Verification items for the finished model (mm, model axes). A direction names the side the tool comes from. Coordinates: 2 decimals unless noted, no trailing zeros. Order: outer loops, then holes, each group sorted by start corner. A loop starts at its lowest first (then second) coordinate and runs counter-clockwise, first axis right, second up. Notation, with made-up numbers: M 9,7 L 41,7 A10 cw 41,22 Z; hole C -22.75,-21.5 d5. An arc over 180 degrees is marked long. Write item = value, one per line.
```python
from build123d import *

# Parameters (mm, degrees)
CHAMFER1_SIZE      = 1
CHAMFER2_SIZE      = 2
SKETCH2_OUTSIDE_W  = 33.844
SKETCH2_OUTSIDE_H  = 33.844
CUT_EXTRUDE1_DEPTH = 6


with BuildPart() as part:
    # Sketch1 → Revolve1 (revolve)
    with BuildSketch(Plane.XY, mode=Mode.PRIVATE) as revolve1_sk:
        with BuildLine():
            Line((87, 0), (87, 3))
            Line((87, 3), (79, 3))
            Line((79, 3), (79, 5))
            Line((79, 5), (25, 5))
            Line((25, 5), (25, 7))
            Line((25, 7), (13, 7))
            Line((13, 7), (13, 5))
            Line((13, 5), (10, 5))
            Line((10, 5), (10, 4))
            Line((10, 4), (3, 4))
            Line((3, 4), (3, 5))
            Line((3, 5), (1.310723572, 5))
            ThreePointArc((1.310723572, 5), (0.382949383, 2.571411472), (0, 0))
            Line((0, 0), (87, 0))
        make_face()
    revolve(revolve1_sk.sketch.rotate(Axis((0, 0, 0), (1, 0, 0)), 90), axis=Axis((0, 0, 0), (1, 0, 0)))

    # Chamfer1
    chamfer1_edges = [part.edges().sort_by_distance(p)[0] for p in [
        (87, 0, -3),
    ]]
    chamfer(chamfer1_edges, length=CHAMFER1_SIZE)

    # Chamfer2
    chamfer2_edges = [part.edges().sort_by_distance(p)[0] for p in [
        (13, 0, -7),
        (25, 0, -5),
    ]]
    chamfer(chamfer2_edges, length=CHAMFER2_SIZE - 0.0001)  # a hair under: the kernel refuses the full size

    # Sketch2 outside → Cut-Extrude1 (cut)
    with BuildSketch(Plane(origin=(79, 0, 0), x_dir=(0, 0, -1), z_dir=(1, 0, 0))):
        Rectangle(SKETCH2_OUTSIDE_W, SKETCH2_OUTSIDE_H)
        Polygon((0, 5.656854249), (5.656854249, 0), (0, -5.656854249), (-5.656854249, 0), align=None, mode=Mode.SUBTRACT)
    extrude(amount=-CUT_EXTRUDE1_DEPTH, mode=Mode.SUBTRACT)


solid = part.part
```
Item 1: Sectioned sample at B-B, the plane x = 82. Enter the section's corners in (y, z).
Report:
outline = C 0,0 d6
Item 2: Scan lines: L1, parallel to Z at x = 34, y = -0.75; L2, parallel to Y at x = 9.5, z = 0; L3, parallel to X at y = -1.75, z = -4. Record each from-to range of solid material in increasing order. Write a range as from..to.
Report:
L1 = -4.94..4.94
L2 = -4..4
L3 = 1.01..3, 10..73
Item 3: Tool access check on faces 1 (the flat face through (76.042, -2.799, -2.858)), 2 (the cylindrical face through (2, 0, -5)), 3 (the flat face through (73, 3, 3)). Record the directions out of +Z, -Z, +X, -X, +Y, -Y that give a thin tool (end or side, any length) a straight path to the whole face; none if there is none.
Report:
face_1 = -Z, +X, -Y
face_2 = -X
face_3 = +Z, +X, +Y
Item 4: Sectioned sample at A-A, the plane x = 72. Enter the section's corners in (y, z), then the cut area to 3 significant figures.
Report:
outline = C 0,0 d10
area = 78.5 mm^2
Item 5: Release check for a two-part mould opening along X. For faces 4 (the cylindrical face through (6.451, 3.905, -0.867)), 5 (the flat face through (79, 3.3, 0.1)), 6 (the cylindrical face through (19.93, 6.21, 3.23)) record: pulls with the +X half, pulls with the -X half, needs draft (parallel to the pull), parting line crosses it, or undercut.
Report:
face_4 = undercut
face_5 = pulls with the +X half
face_6 = needs draft
Item 6: Gauge pin test, flat ends, axial feed: pin 1 (1 mm diameter, centred on x = 61.5, z = -3.5, fed in from -Y); pin 2 (2 mm diameter, centred on y = -2, z = 3.5, fed in from +X); pin 3 (1 mm diameter, centred on x = 67.5, y = 0.5, fed in from +Z). Record the tip position at first contact, or that the pin passes through.
Report:
pin_1 = -4
pin_2 = 79
pin_3 = 5
